Build history of the part. All positions in model axes, mm. Round coordinates to 2 decimals unless told otherwise and drop trailing zeros. Order: outer loops, then holes, each group sorted by start corner. A loop starts at its lowest first (then second) coordinate and runs counter-clockwise, first axis right, second up. Notation, with made-up numbers: M 65,-7 L 106,-7 A21 cw 106,23 Z; hole C -27,18.25 d4. An arc over 180 degrees is marked long. One line per item, written item: value. Start each with the question number.
Item 1: Pin check, flat tips, straight feed: pin 1 (4 mm diameter, centred on x = -125.36, y = -41.985, fed in from -Z); pin 2 (2 mm diameter, centred on x = -83.375, y = 21.5, fed in from +Z). Stop position of each tip, or through.
Item 2: Band-saw the part on A-A, the plane y = 0. Write the cut outline in (x, z), then the cut area to 3 significant figures.
Item 3: Probe L1, parallel to Y at x = -41.39, z = 11.25; L2, parallel to Y at x = -12.7, z = 11; L3, parallel to X at y = 20.5, z = 12. List the from-to ranges inside material, lowest first.
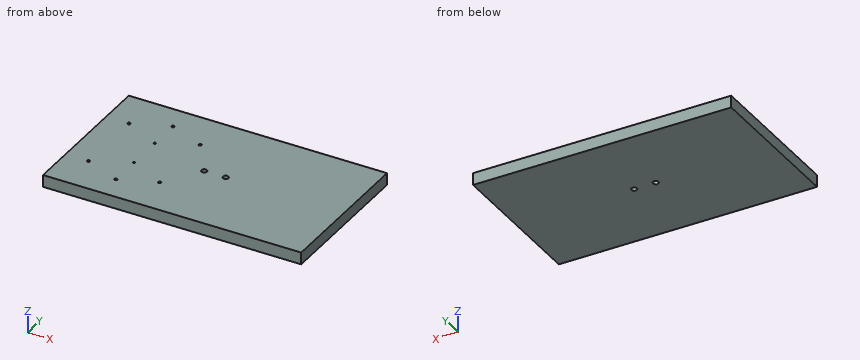
```python
from build123d import *

# Parameters (mm, degrees)
SKETCH1_W                     = 304.8
SKETCH1_H                     = 177.8
BOSS_EXTRUDE1_DEPTH           = 14.224
TAP_DRILL_FOR_8_32_TAP1_D     = 3.4544
TAP_DRILL_FOR_8_32_TAP1_DEPTH = 7.874
TAP_DRILL_FOR_8_32_TAP1_TIP   = 1.037806461
TAP_DRILL_FOR_5_40_TAP1_D     = 2.5781
TAP_DRILL_FOR_5_40_TAP1_DEPTH = 7.874
TAP_DRILL_FOR_5_40_TAP1_TIP   = 0.774539381
F_1_4_CLEARANCE_HOLE1_D       = 6.5278


with BuildPart() as part:
    # Sketch1 → Boss-Extrude1 (new body)
    with BuildSketch(Plane.XY):
        Rectangle(SKETCH1_W, SKETCH1_H)
    extrude(amount=BOSS_EXTRUDE1_DEPTH)

    # Tap Drill for #8-32 Tap1
    with Locations(Plane.XY.offset(14.224)):
        with Locations((-41.39, 41.985), (-41.39, -41.985), (-125.36, -41.985), (-125.36, 41.985), (-83.375, 59.2455), (-83.375, -59.2455)):
            Hole(TAP_DRILL_FOR_8_32_TAP1_D / 2, depth=TAP_DRILL_FOR_8_32_TAP1_DEPTH)
            with Locations((0, 0, -(TAP_DRILL_FOR_8_32_TAP1_DEPTH + TAP_DRILL_FOR_8_32_TAP1_TIP / 2))):  # 118° drill point
                Cone(0, TAP_DRILL_FOR_8_32_TAP1_D / 2, TAP_DRILL_FOR_8_32_TAP1_TIP, mode=Mode.SUBTRACT)

    # Tap Drill for #5-40 Tap1
    with Locations(Plane.XY.offset(14.224)):
        with Locations((-83.375, 21.5), (-83.375, -21.5)):
            Hole(TAP_DRILL_FOR_5_40_TAP1_D / 2, depth=TAP_DRILL_FOR_5_40_TAP1_DEPTH)
            with Locations((0, 0, -(TAP_DRILL_FOR_5_40_TAP1_DEPTH + TAP_DRILL_FOR_5_40_TAP1_TIP / 2))):  # 118° drill point
                Cone(0, TAP_DRILL_FOR_5_40_TAP1_D / 2, TAP_DRILL_FOR_5_40_TAP1_TIP, mode=Mode.SUBTRACT)

    # 1/4 Clearance Hole1 (through all)
    with Locations(Plane(origin=(0, 0, 0), x_dir=(1, 0, 0), z_dir=(0, 0, -1))):
        with Locations((-12.7, 0), (12.7, 0)):
            Hole(F_1_4_CLEARANCE_HOLE1_D / 2)


solid = part.part
```
Output:
1. pin 1: stops at z = 0
1. pin 2: stops at z = 6.18
2. outline: M -152.4,0 L -15.96,0 L -15.96,14.22 L -152.4,14.22 Z; M -9.44,0 L 9.44,0 L 9.44,14.22 L -9.44,14.22 Z; M 15.96,0 L 152.4,0 L 152.4,14.22 L 15.96,14.22 Z
2. area: 4,150 mm²
3. L1: y = -88.9 to -43.71, -40.26 to 40.26, 43.71 to 88.9
3. L2: y = -88.9 to -3.26, 3.26 to 88.9
3. L3: x = -152.4 to -84.19, -82.56 to 152.4
